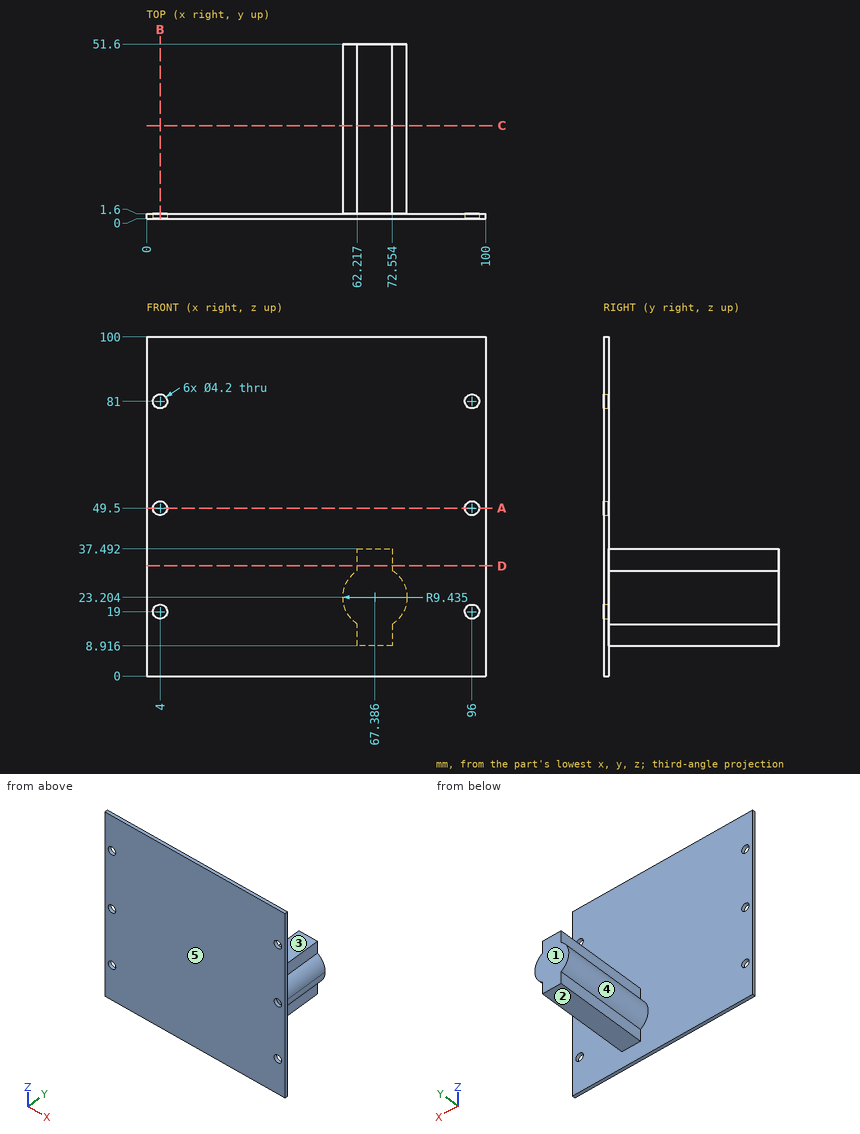
The figure shows three views and two pictorial views of one solid part (mm, origin at its lowest corner). Answer the questions. A direction names the side the tool comes from. Coordinates: 2 decimals unless noted, no trailing zeros. Write each loop counter-clockwise with the first axis right and the second up, starting at its lowest first coordinate (ties: lowest second). Pieces come first, ordered by that corner, then holes. Notation, with made-up numbers: M 64.5,-1.5 L 91.5,-1.5 A25 cw 91.5,30.5 Z; hole C 18,59 d4. An arc over 180 degrees is marked long. Answer as CSV lines item,"result". Start each with the question number.
Item 1: A tool of negligible diameter and unlimited length cuts with its end or side. For the marked faces 1, 2, 3, 4 and 5, from which of +Z, -Z, +X, -X, +Y, -Y can it reach the whole face along a straight path? Write none if from no direction.
Item 2: Section D-D on z = 32.5 is taken. Write down the section's boundary in (x, y), and give its area (3 significant figures).
Item 3: Section B-B on x = 4 is taken. Write down the section's boundary in (y, z), and give its area (3 significant figures).
Item 4: Consider L1, parallel to X at y = 0.8, z = 49.5; L2, parallel to X at y = 16, z = 23; L3, parallel to Y at x = 16.5, z = 22.5. Determine where each line is inside the solid, lowest interval first.
Item 5: Section A-A on z = 49.5 is taken. Write down the section's boundary in (x, y).
Item 6: Flat-ended cylindrical pins translate along their axes: P1, Ø2, axis at x = 36, z = 57.5, coming from the -Y side; P2, Ø5, axis at x = 66, y = 27.5, coming from the -Z side (1 decimal); P3, Ø7, axis at y = 38, z = 33, coming from the -X side; P4, Ø1.9, axis at y = 36, z = 35.5, coming from the +X side. Find the tip coordinate at first contact, or state that the pin passes through.
Item 7: Section C-C on y = 27.5 is taken. Write down the section's boundary in (x, z) (1 decimal).
Checks:
1,face 1,"+Z, -Z, +X, -X, +Y"
1,face 2,"-Z, +X, -X, +Y"
1,face 3,"+Z, +X, -X, +Y"
1,face 4,"-X, +Y"
1,face 5,"+Z, -Z, +X, -X, -Y"
2,outline,"M 0,0 L 100,0 L 100,1.6 L 72.55,1.6 L 72.55,51.6 L 62.22,51.6 L 62.22,1.6 L 0,1.6 Z"
2,area,"677 mm²"
3,outline,"M 0,0 L 1.6,0 L 1.6,16.9 L 0,16.9 Z; M 0,21.1 L 1.6,21.1 L 1.6,47.4 L 0,47.4 Z; M 0,51.6 L 1.6,51.6 L 1.6,78.9 L 0,78.9 Z; M 0,83.1 L 1.6,83.1 L 1.6,100 L 0,100 Z"
3,area,"140 mm²"
4,L1,"x = 0 to 1.9, 6.1 to 93.9, 98.1 to 100"
4,L2,"x = 57.95 to 76.82"
4,L3,"y = 0 to 1.6"
5,outline,"M 0,0 L 1.9,0 L 1.9,1.6 L 0,1.6 Z; M 6.1,0 L 93.9,0 L 93.9,1.6 L 6.1,1.6 Z; M 98.1,0 L 100,0 L 100,1.6 L 98.1,1.6 Z"
6,P1,"stops at y = 0"
6,P2,"stops at z = 8.9"
6,P3,"stops at x = 60.36"
6,P4,"stops at x = 72.55"
7,outline,"M 62.2,8.9 L 72.6,8.9 L 72.6,15.3 A9.4 ccw 72.6,31.1 L 72.6,37.5 L 62.2,37.5 L 62.2,31.1 A9.4 ccw 62.2,15.3 Z"
